Autodesk Inventor part; units mm, degrees
ref_plane "YZ Plane" through (0, 0, 0) normal (1, 0, 0) x (0, 1, 0)
ref_plane "XZ Plane" through (0, 0, 0) normal (0, 1, 0) x (-1, 0, 0)
ref_plane "XY Plane" through (0, 0, 0) normal (0, 0, 1) x (1, 0, 0)
sketch "Sketch1" plane through (0, 0, 0) normal (0, 0, 1) x (1, 0, 0)
  point P0 (0, 0)
sketch "Sketch2" plane through (0, 0, 0) normal (0, 0, 1) x (1, 0, 0)
  line L0 (-15, 113.5) -> (15, 113.5)
  line L1 (15, 113.5) -> (15, 50)
  line L2 (15, 50) -> (-15, 50) construction
  line L3 (-15, 50) -> (-15, 113.5)
  circle A0 centre (0, 0) radius 5 construction
  line L4 (-15, 50) -> (-4.9047, -0.9714)
  line L5 (15, 50) -> (4.9047, -0.9714)
  arc A1 (-4.9047, -0.9714) -> (4.9047, -0.9714) centre (0, 0) ccw
  point P0 (0, 50)
  dimension "d0" = 30
  dimension "d1" = 63.5
  dimension "d2" = 10
  dimension "d3" = 50
extrude "Extrusion1" add sketch "Sketch2" along normal blind 5
sketch "Sketch3" plane through (0, 0, 5) normal (0, 0, 1) x (1, 0, 0)
  line L0 (-10, 108.5) -> (10, 108.5) construction
  line L1 (10, 108.5) -> (10, 55) construction
  line L2 (10, 55) -> (-10, 55) construction
  line L3 (-10, 55) -> (-10, 108.5) construction
  line L4 (15, 113.5) -> (-15, 113.5) construction
  circle A0 centre (-5, 106) radius 2.25
  circle A1 centre (5, 106) radius 2.25
  circle A2 centre (-5, 57.5) radius 2.25
  circle A3 centre (5, 57.5) radius 2.25
  line L5 (-10, 61.5) -> (10, 61.5)
  line L6 (10, 61.5) -> (10, 102)
  line L7 (10, 102) -> (-10, 102)
  line L8 (-10, 102) -> (-10, 61.5)
  line L9 (0, 108.5) -> (0, 55) construction
  point P0 (0, 0)
  point P1 (-10, 81.75)
  point P2 (10, 81.75)
  point P3 (0, 81.75)
  dimension "d6" = 20
  dimension "d7" = 53.5
  dimension "d8" = 5
  dimension "d9" = 4.5
  dimension "d11" = 2.75
  dimension "d12" = 2.5
  dimension "d13" = 2.75
  dimension "d14" = 2.5
  dimension "d15" = 40.5
extrude "Extrusion2" cut sketch "Sketch3" against normal up to next
equation "\"d0\" = s_depth + 2 * b_mat_thickness"
equation "\"d1\" = 2 * s_land + s_width + 2 * b_mat_thickness"
equation "\"d4\" = b_mat_thickness"
equation "\"d6\" = s_depth"
equation "\"d7\" = s_width + 2 * s_land"
equation "\"d8\" = b_mat_thickness"
equation "\"d9\" = s_hole_dia"
equation "\"d11\" = s_hole_side_dist"
equation "\"d12\" = s_hole_front_dist"
equation "\"d13\" = s_hole_side_dist"
equation "\"d14\" = s_hole_front_dist"
equation "\"d15\" = s_width"
equation "\"d16\" = b_mat_thickness"
properties part number "Lower_leg"
Can you work these out from the model? Positions are in its coordinate system, mm. A direction names the side the tool comes from. Give positions to 0.01 mm unless a question says otherwise; leave off trailing zeros. Loops run counter-clockwise (first coordinate to the right, second up) from the corner with the lowest first, then second, coordinate; pieces in that order, holes last. Notation, with made-up numbers: M -16.5,-10.5 L 41.5,-10.5 A24 ccw 41.5,13.5 Z; hole C -40,46 d7. An arc over 180 degrees is marked long. One line per item, written item: value. Start each with the question number.
1) If we section it at D-D, the plane x = -0.25: Write out the boundary of the cut face in (y, z), and give its area (3 significant figures).
2) If we section it at C-C, the plane z = 0.75: Write out the boundary of the cut face in (x, y).
3) Thinking about a two-plate mould opening in X: for faces 3 (the face through (15, 82, 2)), 4 (the face through (0, -5, 2)), 5 (the face through (0, 102, 3)), 6 (the face through (0, 113.5, 2)), which applies, +X half, -X half, draft (parallel to the pull), parting line (faces both ways), or undercut?
4) I'm going to push flat-ended pins straight in: pin 1 (4 mm diameter, centred on x = 5, y = 106, fed in from -Z); pin 2 (3 mm diameter, centred on y = 12, z = 4.5, fed in from -X); pin 3 (2.5 mm diameter, centred on x = 3.5, z = 3, fed in from -Y). Where does each tip first touch, or does it pass through?
5) If we section it at A-A, the plane y = 57.5: Write out the boundary of the cut face in (x, z).
6) If I drill on line 1 (X direction, y = 65, z = 2.9); line 2 (Y direction, x = -4.5, z = 1.2); line 3 (X direction, y = 105, z = 3.8), over which ranges is the centre line in solid material (lowest first)? Write a range as [from, to].
7) If we section it at B-B, the plane y = 96: Write out the boundary of the cut face in (x, z), and give its area (3 significant figures).
8) On a 3-axis mill with a long thin cutter (end or side, diameter ignored), from which of +Z, -Z, +X, -X, +Y, -Y can I reach the whole of each face in a straight line? I mean faces 1 (the face through (-10.023, 24.871, 2.465)), 2 (the face through (-10, 82, 3)). Say none if no direction works.
Completed:
1. outline: M -4.99,0 L 61.5,0 L 61.5,5 L -4.99,5 Z; M 102,0 L 113.5,0 L 113.5,5 L 102,5 Z
1. area: 390 mm^2
2. outline: M -15,50 L -4.9,-0.97 A5 ccw 4.9,-0.97 L 15,50 L 15,113.5 L -15,113.5 Z; hole M -10,61.5 L 10,61.5 L 10,102 L -10,102 Z; hole C -5,57.5 d4.5; hole C -5,106 d4.5; hole C 5,57.5 d4.5; hole C 5,106 d4.5
3. face 3: +X half
3. face 4: parting line
3. face 5: undercut
3. face 6: draft
4. pin 1: passes through
4. pin 2: stops at x = -7.77
4. pin 3: stops at y = -4.47
5. outline: M -15,0 L -7.25,0 L -7.25,5 L -15,5 Z; M -2.75,0 L 2.75,0 L 2.75,5 L -2.75,5 Z; M 7.25,0 L 15,0 L 15,5 L 7.25,5 Z
6. line 1: x = [-15, -10], [10, 15]
6. line 2: y = [-2.18, 55.31], [59.69, 61.5], [102, 103.81], [108.19, 113.5]
6. line 3: x = [-15, -7.02], [-2.98, 2.98], [7.02, 15]
7. outline: M -15,0 L -10,0 L -10,5 L -15,5 Z; M 10,0 L 15,0 L 15,5 L 10,5 Z
7. area: 50.0 mm^2
8. face 1: +Z, -Z, -X, -Y
8. face 2: +Z, -Z
